Design review of the part built by this model. Coordinates are the model's own, in mm. A direction names the side the tool comes from. Coordinates: 2 decimals unless noted, no trailing zeros. Loops run counter-clockwise (first coordinate to the right, second up) from the corner with the lowest first, then second, coordinate; pieces in that order, holes last. Notation, with made-up numbers: (55.25, 70) -> (83.25, 70) arc R21 ccw to (83.25, 85) -> close; hole circle Ø4 at (-26, 32). An arc over 180 degrees is marked (long way). Answer as a JSON object with one key per item and string values.
```python
from build123d import *

# Parameters (mm, degrees)
PAD007_DEPTH = 7.5
SKETCH022_W  = 5.417957
SKETCH022_H  = 1.6504247125
PAD008_DEPTH = 7.5
PAD009_DEPTH = 1.5


with BuildPart() as part:
    # Sketch021 → Pad007 (new body, symmetric)
    with BuildSketch(Plane.YZ):
        Polygon((0, -11.6652847125), (-13.832417, -11.6652847125), (-15.186558, -3.04616), (-15.186558, 14.3347152875), (0, 14.3347152875), align=None)
    pad007 = extrude(amount=PAD007_DEPTH, both=True)

    # Sketch022 → Pad008 (join)
    with BuildSketch(Plane.YZ):
        with Locations((-2.7089785, 15.1599276438)):
            Rectangle(SKETCH022_W, SKETCH022_H)
    pad008 = extrude(amount=-PAD008_DEPTH)

    # Sketch023 → Pad009 (join, symmetric)
    with BuildSketch(Plane.YZ):
        Polygon((0, 20.079264), (-3.377041, 14.3347152875), (0, 14.3347152875), align=None)
    pad009 = extrude(amount=PAD009_DEPTH, both=True)

    # Mirrored006: Pad007, Pad008, Pad009 across Sketch021 V_Axis
    add(pad007.mirror(Plane(origin=(0, 0, 0), x_dir=(1, 0, 0), z_dir=(0, 1, 0))))
    add(pad008.mirror(Plane(origin=(0, 0, 0), x_dir=(1, 0, 0), z_dir=(0, 1, 0))))
    add(pad009.mirror(Plane(origin=(0, 0, 0), x_dir=(1, 0, 0), z_dir=(0, 1, 0))))


with BuildPart() as part_1:
    # Body003 placement: moved
    add(part.part.moved(Location((-7, 0, -4))))


solid = part_1.part
```
1) Add section C-C, the plane x = -1.75. Give the boundary of the cut face in (y, z).
Completed:
{"outline": "(-15.19, -7.05) -> (-13.83, -15.67) -> (13.83, -15.67) -> (15.19, -7.05) -> (15.19, 10.33) -> (-15.19, 10.33) -> close"}
2) Clearance check with flat-ended pins moving along their axes: pin 1 Ø2 at (x, z) = (-2.5, -8.5) entering from +Y; pin 2 Ø1.3 at (x, z) = (-10.5, 11.5) entering from +Y; pin 3 Ø1.7 at (y, z) = (1, 12.5) entering from +X. State where each tip first meets the part, or that it passes through.
Completed:
{"pin 1": "y = 15.12", "pin 2": "y = 5.42", "pin 3": "x = -5.5"}
3) Add section D-D, the plane z = 13.5. Give the boundary of the cut face in (x, y), and give its area (3 significant figures).
Completed:
{"outline": "(-8.5, -1.52) -> (-5.5, -1.52) -> (-5.5, 1.52) -> (-8.5, 1.52) -> close", "area": "9.10 mm²"}
4) For faces 1 (the flat face through (-11, 5.418, 11)), 2 (the flat face through (-11, -5.418, 11)), 3 (the flat face through (-8.5, 0, 14)), 4 (the flat face through (-7, 4, 11)), 5 (the flat face through (-7, -4, 11)), list the 3-axis set-ups (+Z, -Z, +X, -X, +Y, -Y) from which the entire face can be reached by the end or side of a thin tool; tool diameter is ignored.
Completed:
{"face 1": "+Z, +X, -X, +Y", "face 2": "+Z, +X, -X, -Y", "face 3": "+Z, -X, +Y, -Y", "face 4": "+Z, +X, +Y", "face 5": "+Z, +X, -Y"}
5) Wall thickness on probe 1 along Z at (x, y) = (-6.75, 11); probe 2 along Z at (x, y) = (-13.25, 2); probe 3 along X at (y, z) = (3.5, 10.5): over which ranges is each line inside the solid? List them lowest first.
Completed:
{"probe 1": "-15.67 to 10.33", "probe 2": "-15.67 to 11.99", "probe 3": "-14.5 to -7"}
6) Add section B-B, the plane y = 2. Give the boundary of the cut face in (x, z), and give its area (3 significant figures).
Completed:
{"outline": "(-14.5, -15.67) -> (0.5, -15.67) -> (0.5, 10.33) -> (-5.5, 10.33) -> (-5.5, 12.68) -> (-8.5, 12.68) -> (-8.5, 11.99) -> (-14.5, 11.99) -> close", "area": "407 mm²"}
7) Add section A-A, the plane x = -7.75. Give the boundary of the cut face in (y, z).
Completed:
{"outline": "(-15.19, -7.05) -> (-13.83, -15.67) -> (13.83, -15.67) -> (15.19, -7.05) -> (15.19, 10.33) -> (5.42, 10.33) -> (5.42, 11.99) -> (2.41, 11.99) -> (0, 16.08) -> (-2.41, 11.99) -> (-5.42, 11.99) -> (-5.42, 10.33) -> (-15.19, 10.33) -> close"}
